Part model, mm, in its own coordinate system. A direction names the side the tool comes from. Give positions to 0.01 mm unless a question says otherwise; leave off trailing zeros. Order: outer loops, then holes, each group sorted by start corner. A loop starts at its lowest first (then second) coordinate and runs counter-clockwise, first axis right, second up. Notation, with made-up numbers: (3.25, -14.75) - (35.25, -14.75) arc R29 ccw to (35.25, 13.25) - close; hole circle Ø11 at (65.25, -17.75). An arc over 180 degrees is marked (long way). One line per item, written item: value.
```python
from build123d import *

# Parameters (mm, degrees)
SKETCH1_W           = 50.8
SKETCH1_H           = 25.4
BOSS_EXTRUDE1_DEPTH = 3.81
SKETCH2_W           = 50.8
SKETCH2_H           = 5.08
BOSS_EXTRUDE2_DEPTH = 25.4
CUT_EXTRUDE1_DEPTH  = 25.4
FILLET1_R           = 5.08
FILLET2_R           = 2.54
FILLET3_R           = 2.54


with BuildPart() as part:
    # Sketch1 → Boss-Extrude1 (new body)
    with BuildSketch(Plane(origin=(0, 0, 0), x_dir=(1, 0, 0), z_dir=(0, 1, 0))):
        with Locations((29.828717949, 2.800512821)):
            Rectangle(SKETCH1_W, SKETCH1_H)
    extrude(amount=BOSS_EXTRUDE1_DEPTH)

    # Sketch2 → Boss-Extrude2 (add)
    with BuildSketch(Plane(origin=(0, 3.81, 0), x_dir=(1, 0, 0), z_dir=(0, 1, 0))):
        with Locations((29.828717949, 2.800512821)):
            Rectangle(SKETCH2_W, SKETCH2_H)
    extrude(amount=BOSS_EXTRUDE2_DEPTH)

    # Sketch3 → Cut-Extrude1 (cut)
    with BuildSketch(Plane(origin=(0, 0, -5.340512821), x_dir=(-1, 0, 0), z_dir=(0, 0, -1))):
        with BuildLine():
            ThreePointArc((-6.968717949, 23.114), (-9.508717949, 25.654), (-12.048717949, 23.114))
            Line((-12.048717949, 23.114), (-6.968717949, 23.114))
        make_face()
        with BuildLine():
            Line((-6.968717949, 23.114), (-12.048717949, 23.114))
            ThreePointArc((-12.048717949, 23.114), (-9.508717949, 20.574), (-6.968717949, 23.114))
        make_face()
        with BuildLine():
            ThreePointArc((-19.668717949, 23.114), (-22.208717949, 25.654), (-24.748717949, 23.114))
            Line((-24.748717949, 23.114), (-19.668717949, 23.114))
        make_face()
        with BuildLine():
            Line((-19.668717949, 23.114), (-24.748717949, 23.114))
            ThreePointArc((-24.748717949, 23.114), (-22.208717949, 20.574), (-19.668717949, 23.114))
        make_face()
        with BuildLine():
            ThreePointArc((-37.448717949, 23.114), (-34.908717949, 20.574), (-32.368717949, 23.114))
            Line((-32.368717949, 23.114), (-37.448717949, 23.114))
        make_face()
        with BuildLine():
            Line((-37.448717949, 23.114), (-32.368717949, 23.114))
            ThreePointArc((-32.368717949, 23.114), (-34.908717949, 25.654), (-37.448717949, 23.114))
        make_face()
        with BuildLine():
            ThreePointArc((-50.148717949, 23.114), (-47.608717949, 20.574), (-45.068717949, 23.114))
            Line((-45.068717949, 23.114), (-50.148717949, 23.114))
        make_face()
        with BuildLine():
            Line((-50.148717949, 23.114), (-45.068717949, 23.114))
            ThreePointArc((-45.068717949, 23.114), (-47.608717949, 25.654), (-50.148717949, 23.114))
        make_face()
    extrude(amount=-CUT_EXTRUDE1_DEPTH, mode=Mode.SUBTRACT)

    # Fillet1
    fillet1_edges = [part.edges().sort_by_distance(p)[0] for p in [
        (4.428717949, 29.21, -2.800512821),
        (55.228717949, 29.21, -2.800512821),
    ]]
    fillet(fillet1_edges, radius=FILLET1_R)

    # Fillet2
    fillet2_edges = [part.edges().sort_by_distance(p)[0] for p in [
        (29.828717949, 3.81, -0.260512821),
        (29.828717949, 3.81, -5.340512821),
    ]]
    fillet(fillet2_edges, radius=FILLET2_R)

    # Fillet3
    fillet3_edges = [part.edges().sort_by_distance(p)[0] for p in [
        (4.428717949, 1.905, -15.500512821),
        (55.228717949, 1.905, -15.500512821),
        (55.228717949, 1.905, 9.899487179),
        (4.428717949, 1.905, 9.899487179),
    ]]
    fillet(fillet3_edges, radius=FILLET3_R)


solid = part.part
```
1) Slice it at B-B on z = 5.25. Write the cut outline in (x, y), then the cut area to 3 significant figures.
Answer:
outline: (4.43, 0) - (55.23, 0) - (55.23, 3.81) - (4.43, 3.81) - close
area: 194 mm2
2) Which spindle directions (+Z, -Z, +X, -X, +Y, -Y) get a long thin tool onto all of the face, cutting with end or side? Do faces 5 (the face through (29, 18, -5.341)), 6 (the face through (30, 29.21, -3)), 7 (the face through (29, 3.81, 6)). Say none if no direction does.
Answer:
face 5: -Z, +X, -X, +Y
face 6: +Z, -Z, +X, -X, +Y
face 7: +Z, +X, -X, +Y
3) Two-plate mould, pull along X, no slides. Class faces 1 (the face through (29, 0, -3)), 2 (the face through (8.958, 25.594, -2.836)), 3 (the face through (54.46, 1.93, 9.18)), 4 (the face through (5.153, 1.932, -14.737)): pulls with the +X half, pulls with the -X half, needs draft (parallel to the pull), parting line crosses it, or undercut.
Answer:
face 1: needs draft
face 2: undercut
face 3: pulls with the +X half
face 4: pulls with the -X half
4) Wall check: line 1 along Y through (x, z) = (33, -9); line 2 along Z through (x, y) = (52, 14.5); line 3 along X through (y, z) = (23.5, -0.5). Give the ranges that are in metal, low to high. Write a range as [from, to].
Answer:
line 1: y = [0, 3.81]
line 2: z = [-5.34, -0.26]
line 3: x = [4.43, 7], [12.02, 19.7], [24.72, 32.4], [37.42, 45.1], [50.12, 55.23]
5) Slice it at A-A on x = 30. Write the cut outline in (y, z).
Answer:
outline: (0, -15.5) - (3.81, -15.5) - (3.81, -7.88) arc R2.54 cw to (6.35, -5.34) - (29.21, -5.34) - (29.21, -0.26) - (6.35, -0.26) arc R2.54 cw to (3.81, 2.28) - (3.81, 9.9) - (0, 9.9) - close
6) Slice it at D-D on x = 51. Write the cut outline in (y, z), then the cut area to 3 significant figures.
Answer:
outline: (0, -15.5) - (3.81, -15.5) - (3.81, -7.88) arc R2.54 cw to (6.35, -5.34) - (29.14, -5.34) - (29.14, -0.26) - (6.35, -0.26) arc R2.54 cw to (3.81, 2.28) - (3.81, 9.9) - (0, 9.9) - close
area: 228 mm2
7) Drop flat-ended pins along their axis: P1, Ø8, axis at x = 34.91, y = 23.11, coming from the +Z side; P2, Ø3, axis at x = 47.61, y = 23.11, coming from the +Z side; P3, Ø8.5, axis at x = 17.5, z = -13, coming from the +Y side. Give the stop position or say it passes through.
Answer:
P1: stops at z = -0.26
P2: passes through
P3: stops at y = 3.81
8) Slice it at C-C on y = 15.25. Write the cut outline in (x, z).
Answer:
outline: (4.43, -5.34) - (55.23, -5.34) - (55.23, -0.26) - (4.43, -0.26) - close
